```python
from build123d import *

# Parameters (mm, degrees)
SKETCH1_R           = 14
BOSS_EXTRUDE1_DEPTH = 11
CUT_EXTRUDE1_START  = -7
SKETCH2_R           = 14
SKETCH2_R_2         = 13
CUT_EXTRUDE1_DEPTH  = 7
CUT_EXTRUDE2_START  = -1
SKETCH3_R           = 13
SKETCH3_R_2         = 11
CUT_EXTRUDE2_DEPTH  = 1
SKETCH4_R           = 9
CUT_EXTRUDE3_DEPTH  = 5
SKETCH5_R           = 5
CUT_EXTRUDE4_DEPTH  = 5


with BuildPart() as part:
    # Sketch1 → Boss-Extrude1 (new body)
    with BuildSketch(Plane.XY):
        Circle(SKETCH1_R)
    extrude(amount=BOSS_EXTRUDE1_DEPTH)

    # Sketch2 → Cut-Extrude1 (cut)
    with BuildSketch(Plane.XY.offset(11).offset(CUT_EXTRUDE1_START)):
        Circle(SKETCH2_R)
        Circle(SKETCH2_R_2, mode=Mode.SUBTRACT)
    extrude(amount=CUT_EXTRUDE1_DEPTH, mode=Mode.SUBTRACT)

    # Sketch3 → Cut-Extrude2 (cut)
    with BuildSketch(Plane.XY.offset(11).offset(CUT_EXTRUDE2_START)):
        Circle(SKETCH3_R)
        Circle(SKETCH3_R_2, mode=Mode.SUBTRACT)
    extrude(amount=CUT_EXTRUDE2_DEPTH, mode=Mode.SUBTRACT)

    # Sketch4 → Cut-Extrude3 (cut)
    with BuildSketch(Plane.XY.offset(11)):
        Circle(SKETCH4_R)
    extrude(amount=-CUT_EXTRUDE3_DEPTH, mode=Mode.SUBTRACT)

    # Sketch5 → Cut-Extrude4 (cut)
    with BuildSketch(Plane(origin=(0, 0, 0), x_dir=(-1, 0, 0), z_dir=(0, 0, -1))):
        Circle(SKETCH5_R)
    extrude(amount=-CUT_EXTRUDE4_DEPTH, mode=Mode.SUBTRACT)

    # Loft1: read off the stored shape, not the designer's step
    # Loft1: loft between two sections, ruled curve by curve
    loft1_from = [
        Edge.make_bspline([(-2.631639621, 1.44030306, 10), (0.248966499, 6.703582302, 10), (5.512245741, 3.822976182, 10), (2.631639621, -1.44030306, 10), (-0.248966499, -6.703582302, 10), (-5.512245741, -3.822976182, 10), (-2.631639621, 1.44030306, 10)], [0, 0, 0, 0, 0.5, 0.5, 0.5, 1, 1, 1, 1], 3, [1, 0.333333333, 0.333333333, 1, 0.333333333, 0.333333333, 1]),
    ]
    loft1_to = [
        Edge.make_bspline([(-5.534018928, 7.097509035, 6), (8.660999143, 18.165546891, 6), (19.729036998, 3.97052882, 6), (5.534018928, -7.097509035, 6), (-8.660999143, -18.165546891, 6), (-19.729036998, -3.97052882, 6), (-5.534018928, 7.097509035, 6)], [0, 0, 0, 0, 0.5, 0.5, 0.5, 1, 1, 1, 1], 3, [1, 0.333333333, 0.333333333, 1, 0.333333333, 0.333333333, 1]),
    ]
    loft1 = Solid(Shell([*[Face.make_surface_from_curves(loft1_from[k], loft1_to[k]) for k in range(1)], Face(Wire(loft1_from)), Face(Wire(loft1_to))]))
    add(loft1)


solid = part.part
```
The model under review builds one solid part; all positions refer to its coordinate system, in mm. A direction names the side the tool comes from. Round coordinates to 2 decimals unless told otherwise and drop trailing zeros. Write each loop counter-clockwise with the first axis right and the second up, starting at its lowest first coordinate (ties: lowest second). Pieces come first, ordered by that corner, then holes.
(1) Mouldability with a two-part tool opening along Y and no side actions: class faces 4 (the cylindrical face through (-2.38, -10.74, 10.49)), 5 (the flat face through (0, 0, 10)), 6 (the flat face through (9.3, -9.3, 4)) as +Y half, -Y half, draft (parallel to the pull), parting line (faces both ways), or undercut.
(2) We need section C-C on x = 10.5. Give the boundary of the cut face in (y, z), and give its area (3 significant figures).
(3) We need section B-B on z = 0.75. Give the boundary of the cut face in (x, y).
(4) Wall thickness on L1, parallel to Y at x = 0, z = 1.55; L2, parallel to Y at x = 0, z = 9.7; L3, parallel to Y at x = 0, z = 8.4: over which ranges is each line inside the solid? List them lowest first.
(5) Machinability: for faces 1 (the cylindrical face through (-10.316, -7.91, 6.958)), 2 (the flat face through (0, 0, 5)), 3 (the flat face through (0, -6, 0)), which of the approach directions +Z, -Z, +X, -X, +Y, -Y give a long, thin tool a straight path to every point of the face, cutting with its end or side? Answer none if there is none.
(6) We need section A-A on y = 12.25. Give the boundary of the cut face in (x, z).
(7) Insertion check: pin 1 (1.5 mm diameter, centred on x = -4, z = 9, fed in from +Y); pin 2 (6 mm diameter, centred on y = 1.5, z = 9, fed in from +X); pin 3 (4 mm diameter, centred on x = 3, y = 7, fed in from -Z); pin 4 (5 mm diameter, centred on x = -1.5, y = 0.5, fed in from -Z). Each pin has a flat end and moves straight along its axis. Give the tip position at first contact, or say it passes through.
(8) We need section D-D on y = -10. Give the boundary of the cut face in (x, z), and give its area (3 significant figures).
Findings below:
1. face 4: parting line
1. face 5: undercut
1. face 6: draft
2. outline: (-9.26, 0) - (9.26, 0) - (9.26, 4) - (7.66, 4) - (7.66, 10) - (3.28, 10) - (3.28, 11) - (-3.28, 11) - (-3.28, 10) - (-7.66, 10) - (-7.66, 4) - (-9.26, 4) - close
2. area: 173 mm2
3. outline: circle Ø28 at (0, 0); hole circle Ø10 at (0, 0)
4. L1: y = -14 to -5, 5 to 14
4. L2: y = -13 to -9, -3.41 to 3.41, 9 to 13
4. L3: y = -13 to -9, -5.3 to 5.3, 9 to 13
5. face 1: +Z
5. face 2: -Z
5. face 3: -Z, +X, -X, +Y, -Y
6. outline: (-6.78, 0) - (6.78, 0) - (6.78, 4) - (4.35, 4) - (4.35, 10) - (-4.35, 10) - (-4.35, 4) - (-6.78, 4) - close
7. pin 1: stops at y = 12.59
7. pin 2: stops at x = 13
7. pin 3: stops at z = 0
7. pin 4: stops at z = 5
8. outline: (-9.8, 0) - (9.8, 0) - (9.8, 4) - (8.31, 4) - (8.31, 10) - (4.58, 10) - (4.58, 11) - (-4.58, 11) - (-4.58, 10) - (-8.31, 10) - (-8.31, 4) - (-9.8, 4) - close
8. area: 187 mm2
